Geometry check sheet. Reference: the model listing, model coordinates, mm. A direction names the side the tool comes from. Coordinates: 2 decimals unless noted, no trailing zeros. Write each loop counter-clockwise with the first axis right and the second up, starting at its lowest first coordinate (ties: lowest second). Pieces come first, ordered by that corner, then holes. Notation, with made-up numbers: M -30.75,-27 L 5.25,-27 A20 ccw 5.25,4 Z; hole C 61.25,59 d9. An arc over 180 degrees is marked long. Put each result on its own line as item: value. Start each with the question number.
1) Cross-section at D-D on y = -6. Record the cut outline in (x, z), plus the area to 3 significant figures.
2) Set-up check for faces 1 (the cylindrical face through (-2, 12, 3)), 2 (the flat face through (-7, -2, 0)): record each of +Z, -Z, +X, -X, +Y, -Y from which the full face is reachable in a straight line by a thin tool's end or side.
3) Cross-section at A-A on x = 0. Record the cut outline in (y, z), plus the area to 3 significant figures.
4) Mould release check, pull along X, two halves, no side actions. Record for faces 3 (the cylindrical face through (-6.466, -2.681, 4.93)), 4 (the flat face through (0, 15, 3)), 5 (the cylindrical face through (-2, -12, 3)): released by +X, released by -X, zero draft, split by the parting line, or undercut.
5) Scan lines: line 1 along Y through (x, z) = (0, 6.75); line 2 along Y through (x, z) = (0, 3.75); line 3 along X through (y, z) = (4.5, 3). Record each from-to range of solid material in increasing order.
6) Cross-section at C-C on y = 0. Record the cut outline in (x, z), plus the area to 3 significant figures.
7) Cross-section at B-B on z = 3. Record the cut outline in (x, y).
8) Gauge pin test, flat ends, axial feed: pin 1 (4 mm diameter, centred on x = -7, z = 7.5, fed in from +Y); pin 2 (6 mm diameter, centred on y = 8, z = 3, fed in from -X); pin 3 (1 mm diameter, centred on x = -0.5, z = 8.5, fed in from +Y). Record the tip position at first contact, or that the pin passes through.
from build123d import *

# Parameters (mm, degrees)
SKETCH1_R                = 10
BOSS_EXTRUDE1_DEPTH      = 10
SKETCH2_R                = 7
CUT_EXTRUDE1_DEPTH       = 18.320508076
BOSS_EXTRUDE3_REACH      = 30.723
BOSS_EXTRUDE3_END_RADIUS = 10
SKETCH4_R                = 2
CHAMFER2_SIZE            = 0.5


with BuildPart() as part:
    # Sketch1 → Boss-Extrude1 (new body)
    with BuildSketch(Plane.XY):
        Circle(SKETCH1_R)
    extrude(amount=BOSS_EXTRUDE1_DEPTH)

    # Sketch2 → Cut-Extrude1 (cut, through all)
    with BuildSketch(Plane(origin=(0, 0, 0), x_dir=(-1, 0, 0), z_dir=(0, 0, -1))):
        Circle(SKETCH2_R)
    extrude(amount=-CUT_EXTRUDE1_DEPTH, mode=Mode.SUBTRACT)

    # Boss-Extrude3: up to this cylinder (the profile starts outside it)
    boss_extrude3_end = Plane(origin=(0, 0, 3), z_dir=(0, 0, -1)) * Cylinder(BOSS_EXTRUDE3_END_RADIUS, 82.446, mode=Mode.PRIVATE)
    # Sketch4 → Boss-Extrude3 (add, up to the surface)
    with BuildSketch(Plane(origin=(0, 15, 0), x_dir=(1, 0, 0), z_dir=(0, 1, 0)), mode=Mode.PRIVATE) as boss_extrude3_sk1:
        with Locations(Location((0, -3, 0), (0, 0, 270))):
            Circle(SKETCH4_R)
    boss_extrude3_tool1 = extrude(boss_extrude3_sk1.sketch, amount=-BOSS_EXTRUDE3_REACH, mode=Mode.PRIVATE) - boss_extrude3_end
    boss_extrude3 = boss_extrude3_tool1.solids().sort_by_distance((0, 15, 3))[0]
    add(boss_extrude3)

    # Mirror2: Boss-Extrude3 across plane
    add(boss_extrude3.mirror(Plane.ZX))

    # Chamfer2
    chamfer2_edges = [part.edges().sort_by_distance(p)[0] for p in [
        (0, 15, 1),
        (0, -15, 1),
    ]]
    chamfer(chamfer2_edges, length=CHAMFER2_SIZE)


solid = part.part
Answer key:
1. outline: M -8,0 L -3.61,0 L -3.61,10 L -8,10 Z; M 3.61,0 L 8,0 L 8,10 L 3.61,10 Z
1. area: 87.9 mm²
2. face 1: +Y
2. face 2: -Z, +X, -X, +Y, -Y
3. outline: M -15,1.5 L -14.5,1 L -10,1 L -10,0 L -7,0 L -7,10 L -10,10 L -10,5 L -14.5,5 L -15,4.5 Z; M 7,0 L 10,0 L 10,1 L 14.5,1 L 15,1.5 L 15,4.5 L 14.5,5 L 10,5 L 10,10 L 7,10 Z
3. area: 99.5 mm²
4. face 3: undercut
4. face 4: zero draft
4. face 5: split by the parting line
5. line 1: y = -10 to -7, 7 to 10
5. line 2: y = -15 to -7, 7 to 15
5. line 3: x = -8.93 to -5.36, 5.36 to 8.93
6. outline: M -10,0 L -7,0 L -7,10 L -10,10 Z; M 7,0 L 10,0 L 10,10 L 7,10 Z
6. area: 60.0 mm²
7. outline: M -2,-14.5 L -1.5,-15 L 1.5,-15 L 2,-14.5 L 2,-9.8 A10 ccw 2,9.8 L 2,14.5 L 1.5,15 L -1.5,15 L -2,14.5 L -2,9.8 A10 ccw -2,-9.8 Z; hole C 0,0 d14
8. pin 1: stops at y = 8.66
8. pin 2: stops at x = -8.66
8. pin 3: stops at y = 10
